Here's how the part is built. I have some questions about the finished solid (model axes, mm). Coordinates: 2 decimals unless noted, no trailing zeros. Write each loop counter-clockwise with the first axis right and the second up, starting at its lowest first coordinate (ties: lowest second). Pieces come first, ordered by that corner, then holes. Notation, with made-up numbers: (35.25, -39.75) -> (70.25, -39.75) arc R15 ccw to (70.25, -32.75) -> close; hole circle Ø7 at (1.5, 67.5). An arc over 180 degrees is marked (long way). Put each result on its own line as item: value.
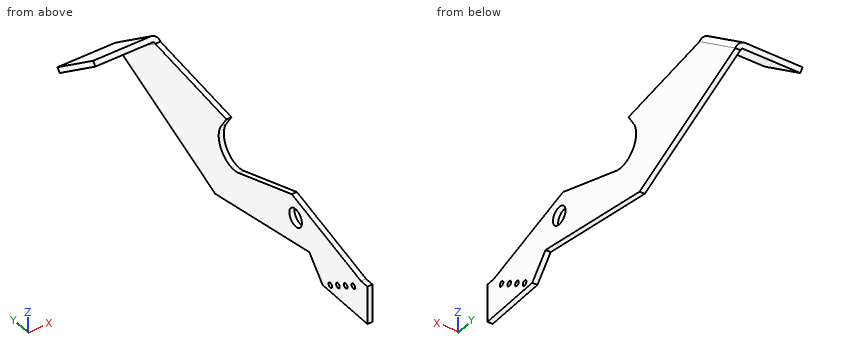
```python
from build123d import *

# Parameters (mm, degrees)
SKETCH_6_R             = 7
SKETCH_6_R_2           = 2
SM_BASE_FLANGE_2_DEPTH = 4
SM_EDGE_FLANGE_1_DEPTH = 50


# Sheet-metal steps are written as plain solids
with BuildPart() as part:
    # Эскиз6 → Базовая кромка2 (new body)
    with BuildSketch(Plane(origin=(0, 0, 0), x_dir=(0, 0, -1), z_dir=(1, 0, 0))):
        with BuildLine():
            Line((-41.515639953, 156.639911011), (-30.570860008, 77.324503301))
            Line((-30.570860008, 77.324503301), (-21.473166605, 83.200308456))
            ThreePointArc((-21.473166605, 83.200308456), (-1.78992877, 82.320794398), (3.842668301, 63.440189352))
            Line((3.842668301, 63.440189352), (-16.29997452, 4.284628471))
            Line((-16.29997452, 4.284628471), (5, -72.987711453))
            Line((5, -72.987711453), (5, -80.109264525))
            Line((5, -80.109264525), (35, -80.109264525))
            Line((35, -80.109264525), (35, -30.109264525))
            Line((35, -30.109264525), (17.952200663, -15.286686185))
            Line((17.952200663, -15.286686185), (37, 89.665096307))
            Line((37, 89.665096307), (-11.325084854, 196.496282933))
            Line((-11.325084854, 196.496282933), (-41.515639953, 156.639911011))
        make_face()
        Circle(SKETCH_6_R, mode=Mode.SUBTRACT)
        with Locations((29.855042446, -38.684193782)):
            Circle(SKETCH_6_R_2, mode=Mode.SUBTRACT)
        with Locations((24.710084891, -47.259123039)):
            Circle(SKETCH_6_R_2, mode=Mode.SUBTRACT)
        with Locations((19.565127337, -55.834052297)):
            Circle(SKETCH_6_R_2, mode=Mode.SUBTRACT)
        with Locations((14.420169783, -64.408981554)):
            Circle(SKETCH_6_R_2, mode=Mode.SUBTRACT)
    extrude(amount=-SM_BASE_FLANGE_2_DEPTH)

    # Ребро-кромка1 section (across the edge) → Ребро-кромка1 (add)
    with BuildSketch(Plane(origin=(-4, 157.545627664, 42.711331111), x_dir=(-3.4914813388431334e-15, -0.6038111019965894, -0.7971274384348241), z_dir=(0, 0.7971274384348241, -0.6038111019965894))):
        with BuildLine():
            Line((-4, 1.5), (-4, 46))
            Line((-4, 46), (0, 46))
            Line((0, 46), (0, 1.5))
            ThreePointArc((0, 1.5), (0.439339828, 0.439339828), (1.5, 0))
            Line((1.5, 0), (1.5, -4))
            ThreePointArc((1.5, -4), (-2.389087297, -2.389087297), (-4, 1.5))
        make_face()
    extrude(amount=SM_EDGE_FLANGE_1_DEPTH)


solid = part.part
```
Item 1: Imagine slicing it at C-C on x = -17.5. Write out the boundary of the cut face in (y, z), then the cut area to 3 significant figures.
Output:
outline: (157.55, 42.71) -> (197.4, 12.52) -> (199.82, 15.71) -> (159.96, 45.9) -> close
area: 200 mm²
Item 2: Imagine slicing it at D-D on y = 104.5. Write out the boundary of the cut face in (x, z), then the cut area to 3 significant figures.
Output:
outline: (-4, -30.29) -> (0, -30.29) -> (0, 34.32) -> (-4, 34.32) -> close
area: 258 mm²
Item 3: Imagine slicing it at B-B on y = 0. Write out the boundary of the cut face in (x, z).
Output:
outline: (-4, -20.73) -> (0, -20.73) -> (0, -7) -> (-4, -7) -> close; (-4, 7) -> (0, 7) -> (0, 15.12) -> (-4, 15.12) -> close
Item 4: Please list where these lines run through material, in increasing order: line 1 along X through (y, z) = (-36, 3); line 2 along Y through (x, z) = (-31.5, 36); line 3 along Y through (x, z) = (-27, 22). Write a range as from..to.
Output:
line 1: x = -4..0
line 2: y = 166.41..173.03
line 3: y = 184.89..191.51
Item 5: Imagine slicing it at A-A on z = 0. Write out the boundary of the cut face in (x, y).
Output:
outline: (-4, -54.85) -> (0, -54.85) -> (0, -7) -> (-4, -7) -> close; (-4, 7) -> (0, 7) -> (0, 52.15) -> (-4, 52.15) -> close; (-4, 80.71) -> (0, 80.71) -> (0, 171.46) -> (-4, 171.46) -> close
Item 6: For P1, Ø4, axis at y = 130.5, z = 13, coming from the -X side; P2, Ø2, axis at x = -1.5, y = -43.5, coming from the -Z side; P3, Ø6, axis at x = -36.5, z = 36.5, coming from the +Y side, each with a flat end and sliding along its axis, tell me the tip position at first contact or that it passes through.
Output:
P1: stops at x = -4
P2: stops at z = -35
P3: stops at y = 176.33
